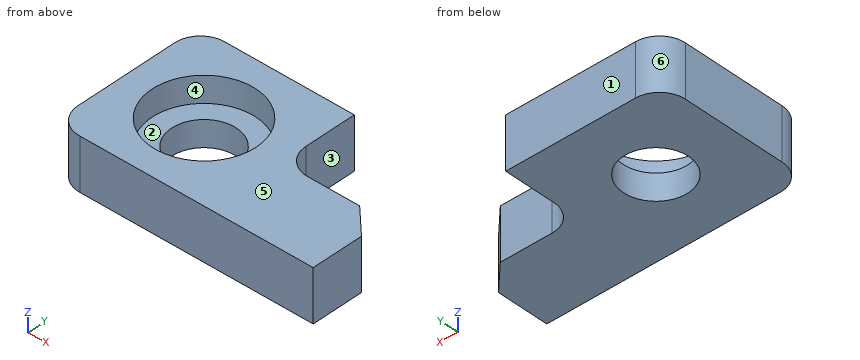
Autodesk Inventor part; units mm, degrees
ref_plane "YZ Plane" through (0, 0, 0) normal (1, 0, 0) x (0, 1, 0)
ref_plane "XZ Plane" through (0, 0, 0) normal (0, 1, 0) x (-1, 0, 0)
ref_plane "XY Plane" through (0, 0, 0) normal (0, 0, 1) x (1, 0, 0)
sketch "Sketch1" plane through (0, 0, 0) normal (0, 0, 1) x (1, 0, 0)
  line L0 (0, 0) -> (100, 0)
  line L1 (100, 0) -> (100, 30)
  line L2 (100, 30) -> (60, 30)
  line L3 (60, 30) -> (60, 60)
  line L4 (60, 60) -> (0, 60)
  line L5 (0, 60) -> (0, 0)
  dimension "d14" = 100
  dimension "d15" = 30
  dimension "d16" = 60
  dimension "d19" = 60
extrude "Extrusion1" add sketch "Sketch1" along normal mid plane 20
chamfer "Chamfer1" distance 10 angle 45 1 edges at (100, 30, 0)
fillet "Fillet1" radius 10 1 edges at (60, 30, 0)
fillet "Fillet3" radius 10 1 edges at (0, 60, 0)
fillet "Fillet4" radius 10 1 edges at (0, 0, 0)
sketch "Sketch2" plane through (0, 0, 10) normal (0, 0, 1) x (1, 0, 0)
  circle A0 centre (30, 30) radius 20
  line L0 (10, 0) -> (100, 0)
  line L1 (0, 50) -> (0, 10)
  point P0 (0, 0)
  point P1 (90, 0)
  dimension "d18" = 30
  dimension "d20" = 30
  dimension "d21" = 40
sketch "Sketch3" plane through (0, 0, 10) normal (0, 0, 1) x (1, 0, 0)
  circle A0 centre (30, 30) radius 12.5
  line L0 (0, 50) -> (0, 10)
  line L1 (10, 0) -> (100, 0)
  point P0 (0, 0)
  point P1 (90, 0)
  dimension "d22" = 30
  dimension "d23" = 30
  dimension "d24" = 25
extrude "Extrusion2" cut sketch "Sketch2" against normal blind 10
extrude "Extrusion3" cut sketch "Sketch3" against normal blind 20
Verification items for the finished model (mm, model axes). Face numbers are marked on the shaded views. A direction names the side the tool comes from. Coordinates: 2 decimals unless noted, no trailing zeros. Loops run counter-clockwise (first coordinate to the right, second up) from the corner with the lowest first, then second, coordinate; pieces in that order, holes last. Notation, with made-up numbers: (30.5, 66) - (40.5, 66) arc R16 cw to (40.5, 91) - close; hole circle Ø2 at (61.25, 69). An arc over 180 degrees is marked (long way). Answer as a JSON object with one key per item and string values.
(1) Scan lines: line 1 along Y through (x, z) = (30, -7.75); line 2 along Y through (x, z) = (30, 5.5); line 3 along Z through (x, y) = (22.5, 17). Record each from-to range of solid material in increasing order.
Response:
{"line 1": "y = 0 to 17.5, 42.5 to 60", "line 2": "y = 0 to 10, 50 to 60", "line 3": "z = -10 to 0"}
(2) Mould release check, pull along Y, two halves, no side actions. Record for the marked faces 4, 5 and 6: pulls with the +Y half, pulls with the -Y half, needs draft (parallel to the pull), parting line crosses it, or undercut.
Response:
{"face 4": "undercut", "face 5": "needs draft", "face 6": "pulls with the +Y half"}
(3) Go/stop test with flat-tipped pins: pin 1 Ø6 at (y, z) = (46.5, -3) entering from +X; pin 2 Ø3 at (y, z) = (27.5, 6) entering from +X; pin 3 Ø10 at (x, z) = (79.5, 0) entering from +Y. Record where each tip stops, or that it passes through.
Response:
{"pin 1": "stops at x = 60", "pin 2": "stops at x = 94", "pin 3": "stops at y = 30"}
(4) Cross-section at C-C, the plane y = 27. Record the boundary of the cut face in (x, z), then the cut area to 3 significant figures.
Response:
{"outline": "(0, -10) - (17.87, -10) - (17.87, 0) - (10.23, 0) - (10.23, 10) - (0, 10) - close; (42.13, -10) - (93, -10) - (93, 10) - (49.77, 10) - (49.77, 0) - (42.13, 0) - close", "area": "1,220 mm²"}
(5) Cross-section at A-A, the plane x = 30. Record the boundary of the cut face in (y, z).
Response:
{"outline": "(0, -10) - (17.5, -10) - (17.5, 0) - (10, 0) - (10, 10) - (0, 10) - close; (42.5, -10) - (60, -10) - (60, 10) - (50, 10) - (50, 0) - (42.5, 0) - close"}
(6) Cross-section at B-B, the plane z = 2.5. Record the boundary of the cut face in (x, y).
Response:
{"outline": "(0, 10) arc R10 ccw to (10, 0) - (100, 0) - (100, 20) - (90, 30) - (70, 30) arc R10 cw to (60, 40) - (60, 60) - (10, 60) arc R10 ccw to (0, 50) - close; hole circle Ø40 at (30, 30)"}
(7) Cross-section at D-D, the plane x = 91. Record the boundary of the cut face in (y, z), then the cut area to 3 significant figures.
Response:
{"outline": "(0, -10) - (29, -10) - (29, 10) - (0, 10) - close", "area": "580 mm²"}
(8) Access from +Z, -Z, +X, -X, +Y, -Y to the whole of each face (thin tool, end or side, straight path). Record for the marked faces 1, 2 and 3.
Response:
{"face 1": "+Z, -Z, +X, -X, +Y", "face 2": "+Z", "face 3": "+Z, -Z, +X, +Y"}
